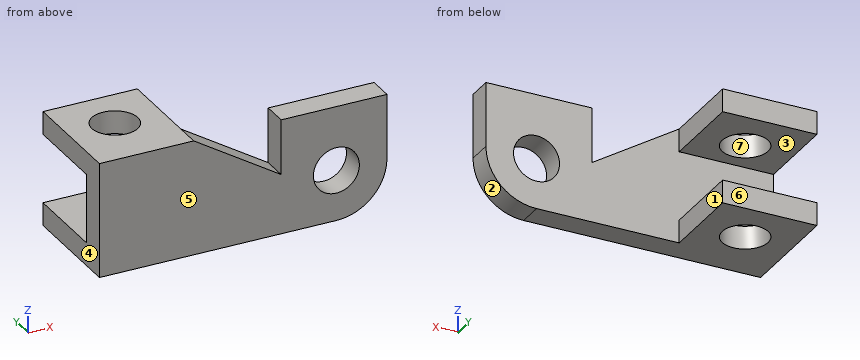
from build123d import *

# Parameters (mm, degrees)
BOSS_EXTRUDE1_DEPTH = 11
SKETCH2_R           = 10
CUT_EXTRUDE1_DEPTH  = 12
SKETCH3_W           = 41
SKETCH3_H           = 10
BOSS_EXTRUDE2_DEPTH = 37
SKETCH4_R           = 10
CUT_EXTRUDE2_DEPTH  = 51
FILLET4_R           = 22


with BuildPart() as part:
    # Sketch1 → Boss-Extrude1 (new body)
    with BuildSketch(Plane(origin=(0, 0, 0), x_dir=(1, 0, 0), z_dir=(0, 1, 0))):
        Polygon((16.5, -25), (62.5, -25), (62.5, 25), (-62.5, 25), (-62.5, -25), (-21.5, -25), (16.5, -1), align=None)
    extrude(amount=BOSS_EXTRUDE1_DEPTH)

    # Sketch2 → Cut-Extrude1 (cut, through all)
    with BuildSketch(Plane(origin=(0, 11, 0), x_dir=(1, 0, 0), z_dir=(0, 1, 0))):
        with Locations((40.5, 3)):
            Circle(SKETCH2_R)
    extrude(amount=-CUT_EXTRUDE1_DEPTH, mode=Mode.SUBTRACT)

    # Sketch3 → Boss-Extrude2 (add)
    with BuildSketch(Plane(origin=(0, 11, 0), x_dir=(1, 0, 0), z_dir=(0, 1, 0))):
        with Locations((-42, 20)):
            Rectangle(SKETCH3_W, SKETCH3_H)
        with Locations((-42, -20)):
            Rectangle(SKETCH3_W, SKETCH3_H)
    extrude(amount=BOSS_EXTRUDE2_DEPTH)

    # Sketch4 → Cut-Extrude2 (cut, through all)
    with BuildSketch(Plane.XY.offset(25)):
        with Locations((-42, 27)):
            Circle(SKETCH4_R)
    extrude(amount=-CUT_EXTRUDE2_DEPTH, mode=Mode.SUBTRACT)

    # Fillet4
    fillet4_edges = [part.edges().sort_by_distance(p)[0] for p in [
        (62.5, 5.5, -25),
    ]]
    fillet(fillet4_edges, radius=FILLET4_R)


solid = part.part
Model file for the job. Use its own axes, mm. Face numbers are marked on the shaded views. A direction names the side the tool comes from. Coordinates: 2 decimals unless noted, no trailing zeros. Write each loop counter-clockwise with the first axis right and the second up, starting at its lowest first coordinate (ties: lowest second). Pieces come first, ordered by that corner, then holes. Notation, with made-up numbers: (-37, 18.5) - (22, 18.5) arc R36 cw to (22, 52.5) - close; hole circle Ø7 at (49.5, 79.25). An arc over 180 degrees is marked (long way). Write each question's results on one line, items separated by ' | '. Start each with the question number.
1) Probe line 1 along Y through (x, z) = (-42, -18); line 2 along X through (y, z) = (4.75, -3); line 3 along Z through (x, y) = (-26.5, 14). List the from-to ranges inside material, lowest first. Write a range as from..to.
2) Cut at D-D (z = -7.5). Write the cut outline in (x, y).
3) Cut at C-C (y = 15.5). Write the cut outline in (x, z), then the cut area to 3 significant figures.
4) 3-axis set-ups, long thin cutter, end or side, ignore diameter. For the marked faces 1, 2 and 3: which of +Z, -Z, +X, -X, +Y, -Y reach the whole face in a straight line?
5) Flat gauge pins, fed straight in: P1, Ø16, axis at x = 40.5, z = -3, coming from the -Y side; P2, Ø8, axis at y = 36.5, z = 18, coming from the +X side. Where does each tip first touch, or does it go through?
6) Cut at A-A (y = 27). Write the cut outline in (x, z), then the cut area to 3 significant figures.
7) Cut at B-B (x = -42). Write the cut outline in (y, z).
8) Mould opens along Y. For the marked faces 4, 5, 6 and 7 say: pulls with the +Y half, pulls with the -Y half, needs draft (parallel to the pull), parting line crosses it, or undercut.
Returned:
1) line 1: 0..17, 37..48 | line 2: -62.5..30.5, 50.5..62.5 | line 3: -25..-15, 15..25
2) outline: (-62.5, 0) - (31.57, 0) - (31.57, 11) - (-62.5, 11) - close; (49.43, 0) - (62.03, 0) - (62.03, 11) - (49.43, 11) - close
3) outline: (-62.5, -25) - (-21.5, -25) - (-21.5, -15) - (-62.5, -15) - close; (-62.5, 15) - (-21.5, 15) - (-21.5, 25) - (-62.5, 25) - close | area: 820 mm^2
4) face 1: +Z, -Z, +X, +Y | face 2: -Z, +X, +Y, -Y | face 3: +X, -X, +Y
5) P1: through | P2: x = -21.5
6) outline: (-62.5, -25) - (-52, -25) - (-52, -15) - (-62.5, -15) - close; (-62.5, 15) - (-52, 15) - (-52, 25) - (-62.5, 25) - close; (-32, -25) - (-21.5, -25) - (-21.5, -15) - (-32, -15) - close; (-32, 15) - (-21.5, 15) - (-21.5, 25) - (-32, 25) - close | area: 420 mm^2
7) outline: (0, -25) - (17, -25) - (17, -15) - (11, -15) - (11, 15) - (17, 15) - (17, 25) - (0, 25) - close; (37, -25) - (48, -25) - (48, -15) - (37, -15) - close; (37, 15) - (48, 15) - (48, 25) - (37, 25) - close
8) face 4: needs draft | face 5: pulls with the -Y half | face 6: pulls with the +Y half | face 7: undercut
